For this review, use the dimensioned drawing (mm, ordinates from the lowest corner) and the shaded views. A direction names the side the tool comes from. Coordinates: 2 decimals unless noted, no trailing zeros. Write each loop counter-clockwise with the first axis right and the second up, starting at its lowest first coordinate (ties: lowest second). Pieces come first, ordered by that corner, then holes. Notation, with made-up numbers: M 82.5,-38 L 122.5,-38 A20 cw 122.5,-1 Z; hole C 22,-6.75 d6. An arc over 180 degrees is marked long. One line per question, with ' | ' between items.
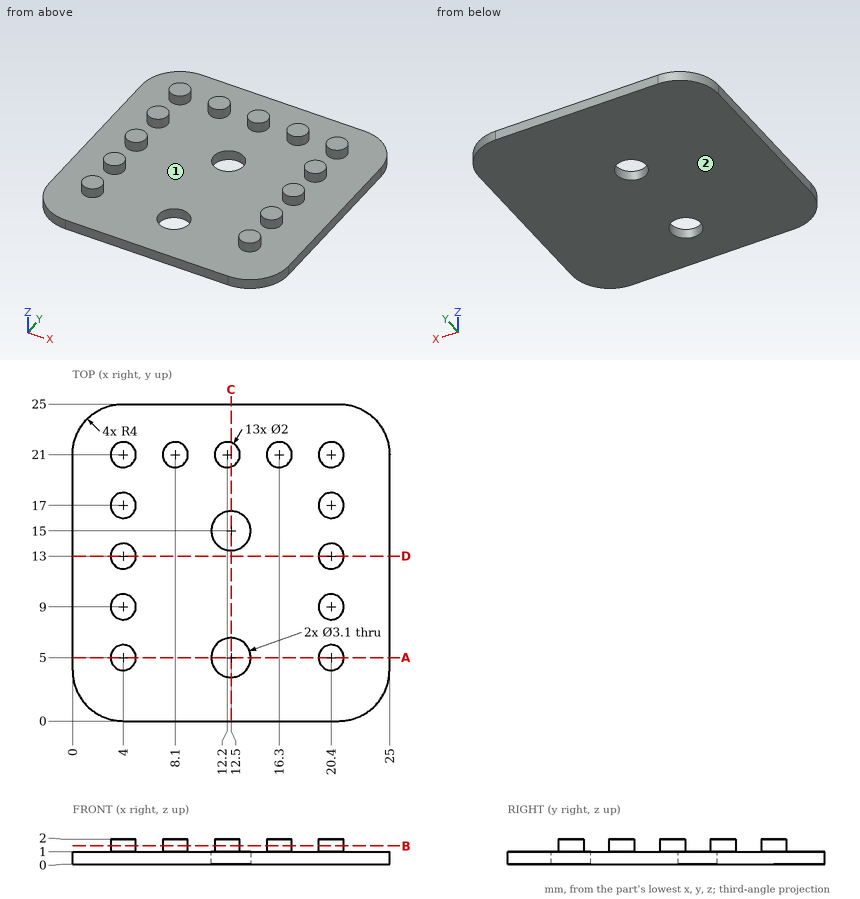
1) We need section D-D on y = 13. State the section outline as (x, z) points.
Responses:
outline: M 0,0 L 25,0 L 25,1 L 21.4,1 L 21.4,2 L 19.4,2 L 19.4,1 L 5,1 L 5,2 L 3,2 L 3,1 L 0,1 Z
2) To check wall thickness, follow line 1 along Y through (x, z) = (12.5, 0.3); line 2 along Z through (x, y) = (22.75, 4); line 3 along X through (y, z) = (22.75, 0.4). State the ranges of each line that lie inside material, in increasing order. Write a range as [from, to].
Responses:
line 1: [0, 3.45], [6.55, 13.45], [16.55, 25] | line 2: [0, 1] | line 3: [0.4, 24.6]
3) We need section B-B on z = 1.45. State how many separate pieces and enclosed holes the cut face has, then the cut area to 3 significant figures.
Responses:
separate pieces: 13 | enclosed holes: 0 | area: 40.8 mm^2
4) We need section C-C on x = 12.5. State the section outline as (y, z) points.
Responses:
outline: M 0,0 L 3.45,0 L 3.45,1 L 0,1 Z; M 6.55,0 L 13.45,0 L 13.45,1 L 6.55,1 Z; M 16.55,0 L 25,0 L 25,1 L 21.95,1 L 21.95,2 L 20.05,2 L 20.05,1 L 16.55,1 Z
5) Machinability: for the marked faces 1 and 2, which of the approach directions +Z, -Z, +X, -X, +Y, -Y give a long, thin tool a straight path to every point of the face, cutting with its end or side? Answer none if there is none.
Responses:
face 1: +Z | face 2: -Z, +X, -X, +Y, -Y
6) We need section A-A on y = 5. State the section outline as (x, z) points, then the cut area to 3 significant figures.
Responses:
outline: M 0,0 L 10.95,0 L 10.95,1 L 5,1 L 5,2 L 3,2 L 3,1 L 0,1 Z; M 14.05,0 L 25,0 L 25,1 L 21.4,1 L 21.4,2 L 19.4,2 L 19.4,1 L 14.05,1 Z | area: 25.9 mm^2
